from build123d import *

# Parameters (mm, degrees)
EXTRUDE_1_DEPTH = 3
FILLET_1_R      = 2


with BuildPart() as part:
    # 草图1 → 凸台-拉伸1 (new body)
    with BuildSketch(Plane(origin=(0, 0, 0), x_dir=(0, 0, -1), z_dir=(1, 0, 0))):
        Polygon((3.5, 5.6), (-3.5, 5.6), (-9.6, -4), (-9.6, -12), (7.6, -12), (7.6, -4), align=None)
        with BuildLine():
            ThreePointArc((-2.59, -9), (-3.595, -10.005), (-4.6, -9))
            Line((-4.6, -9), (-4.6, -6))
            ThreePointArc((-4.6, -6), (-3.595, -4.995), (-2.59, -6))
            Line((-2.59, -6), (1.59, -6))
            ThreePointArc((1.59, -6), (2.595, -4.995), (3.6, -6))
            Line((3.6, -6), (3.6, -9))
            ThreePointArc((3.6, -9), (2.595, -10.005), (1.59, -9))
            Line((1.59, -9), (-2.59, -9))
        make_face(mode=Mode.SUBTRACT)
        with BuildLine():
            ThreePointArc((2.505, -2.095), (2.210642315, -2.805642315), (1.5, -3.1))
            Line((1.5, -3.1), (-1.5, -3.1))
            ThreePointArc((-1.5, -3.1), (-2.505, -2.095), (-1.5, -1.09))
            Line((-1.5, -1.09), (-1.5, 1.09))
            ThreePointArc((-1.5, 1.09), (-2.505, 2.095), (-1.5, 3.1))
            Line((-1.5, 3.1), (1.5, 3.1))
            ThreePointArc((1.5, 3.1), (2.210642315, 2.805642315), (2.505, 2.095))
            ThreePointArc((2.505, 2.095), (2.210642315, 1.384357685), (1.5, 1.09))
            Line((1.5, 1.09), (1.5, -1.09))
            ThreePointArc((1.5, -1.09), (2.210642315, -1.384357685), (2.505, -2.095))
        make_face(mode=Mode.SUBTRACT)
    extrude(amount=EXTRUDE_1_DEPTH)

    # 圆角1
    fillet_1_edges = [part.edges().sort_by_distance(p)[0] for p in [
        (1.5, 5.6, 3.5),
        (1.5, 5.6, -3.5),
        (1.5, -4, -7.6),
        (1.5, -12, -7.6),
        (1.5, -12, 9.6),
        (1.5, -4, 9.6),
    ]]
    fillet(fillet_1_edges, radius=FILLET_1_R)


solid = part.part
Source: CAD feature listing. Evaluate the final solid. Frame: model axes, mm. A direction names the side the tool comes from. Coordinates: 2 decimals unless noted, no trailing zeros. Loops run counter-clockwise (first coordinate to the right, second up) from the corner with the lowest first, then second, coordinate; pieces in that order, holes last. Notation, with made-up numbers: (14.25, -3) - (72.25, -3) arc R27 ccw to (72.25, 17) - close; hole circle Ø7 at (-30, 56.5). An arc over 180 degrees is marked (long way). One line per question, with ' | ' between items.
1) Pull-direction query (Z, two-part tool) for faces 1 (the face through (1.52, -11.4, 9.03)), 2 (the face through (1, -12, 1)), 3 (the face through (1, -7, -7.6)), 4 (the face through (1.479, -10.005, 3.573)); classes: released by +Z, released by -Z, zero draft, split by the parting line, or undercut.
Report:
face 1: released by +Z | face 2: zero draft | face 3: released by -Z | face 4: undercut
2) Set-up query: faces 5 (the face through (1.479, -2.117, 2.505)), 6 (the face through (1.52, -4.02, 9.52)). Return all of +Z, -Z, +X, -X, +Y, -Y with unobstructed straight access to the full face (end or side cutting, diameter ignored); none if empty.
Report:
face 5: +X, -X | face 6: +Z, +X, -X, +Y
3) Line query: line 1 along Y through (x, z) = (1.4, -0.75); line 2 along Y through (x, z) = (2.15, -2); line 3 along Z through (x, y) = (0.9, -8). Output: solid intervals per line, ascending.
Report:
line 1: y = -12 to -9, -6 to -3.1, 3.1 to 5.6 | line 2: y = -12 to -9.81, -5.19 to -2.97, -1.22 to 1.22, 2.97 to 5.6 | line 3: z = -7.6 to -3.6, 4.6 to 9.6
4) First-contact query: P1, Ø1.5, axis at x = 0.5, z = -4.5, coming from the +Y side; P2, Ø1.7, axis at x = 2, y = 0, coming from the +Z side. Flat tips, straight axial feed; report the tip coordinate or a pass-through.
Report:
P1: stops at y = 4.84 | P2: stops at z = 7.6
5) Section D-D, the plane y = 3.5. Return loops of the section in (x, z).
Report:
outline: (0, -4.4) - (3, -4.4) - (3, 4.83) - (0, 4.83) - close
6) Section C-C, the plane z = -1. Return loops of the section in (x, y).
Report:
outline: (0, -12) - (3, -12) - (3, -9) - (0, -9) - close; (0, -6) - (3, -6) - (3, -3.1) - (0, -3.1) - close; (0, 3.1) - (3, 3.1) - (3, 5.6) - (0, 5.6) - close
7) Section A-A, the plane x = 0.55. Return loops of the section in (y, z) (3 decimals), then the cut area to 3 significant figures.
Report:
outline: (-12, -5.6) arc R2 ccw to (-10, -7.6) - (-4.409, -7.6) arc R2 ccw to (-3.624, -7.439) - (4.386, -4.019) arc R2 ccw to (5.6, -2.179) - (5.6, 2.401) arc R2 ccw to (4.673, 4.089) - (-3.509, 9.288) arc R2 ccw to (-4.582, 9.6) - (-10, 9.6) arc R2 ccw to (-12, 7.6) - close; hole (-9, -3.6) - (-6, -3.6) arc R1.005 ccw to (-6, -1.59) - (-6, 2.59) arc R1.005 ccw to (-6, 4.6) - (-9, 4.6) arc R1.005 ccw to (-9, 2.59) - (-9, -1.59) arc R1.005 ccw to start; hole (-3.1, -1.5) arc R1.005 ccw to (-1.09, -1.5) - (1.09, -1.5) arc R1.005 ccw to (3.1, -1.5) - (3.1, 1.5) arc R1.005 ccw to (1.09, 1.5) - (-1.09, 1.5) arc R1.005 ccw to (-3.1, 1.5) - close | area: 196 mm²
8) Section B-B, the plane y = -0.5. Return loops of the section in (x, z), then the cut area to 3 significant figures.
Report:
outline: (0, -6.11) - (3, -6.11) - (3, -1.5) - (0, -1.5) - close; (0, 1.5) - (3, 1.5) - (3, 7.38) - (0, 7.38) - close | area: 31.4 mm²
